For this review, take the finished solid that the model builds, in its own axes (mm). A direction names the side the tool comes from. Coordinates: 2 decimals unless noted, no trailing zeros. One line per item, written item: value. Start each with the question number.
1. Insertion check: pin 1 (1.7 mm diameter, centred on y = -1, z = 328.5, fed in from -X). The pin has a flat end and moves straight along its axis. Give the tip position at first contact, or say it passes through.
2. To check wall thickness, follow line 1 (Y direction, x = 0, z = 22.5); line 2 (Y direction, x = 0.25, z = 302.5); line 3 (Y direction, x = 4, z = 232). State the ranges of each line that lie inside material, in increasing order. Write a range as from..to.
3. For faces 5 (the face through (-3.9, 0, 28)), 6 (the face through (2, 2, 0)), 7 (the face through (3.9, 0, 28)), list the 3-axis set-ups (+Z, -Z, +X, -X, +Y, -Y) from which the entire face can be reached by the end or side of a thin tool; tool diameter is ignored.
4. The part is to be moulded in two halves that separate along Y. For faces 1 (the face through (0.057, -2.843, 56.541)), 2 (the face through (0, -3.9, 177)), 3 (the face through (0, 3.9, 177)), 4 (the face through (3.9, 0, 331)), say which applies: released by +Y, released by -Y, zero draft, split by the parting line, or undercut.
```python
from build123d import *

# Parameters (mm, degrees)
SKETCH_2_R          = 2.55
EXTRUDE_1_DEPTH     = 360
SKETCH_3_R          = 3
CUT_EXTRUDE_1_DEPTH = 361.693775937


with BuildPart() as part:
    # 草图2 → 凸台-拉伸1 (new body)
    with BuildSketch(Plane.XY):
        with BuildLine():
            Line((-3.9, 2.839339828), (-6.560660172, 5.5))
            Line((-6.560660172, 5.5), (-8.2, 5.5))
            Line((-8.2, 5.5), (-8.2, 3.1))
            Line((-8.2, 3.1), (-9.45, 3.1))
            Line((-9.45, 3.1), (-9.45, 3.65))
            Line((-9.45, 3.65), (-10, 3.65))
            Line((-10, 3.65), (-10, 8.5))
            ThreePointArc((-10, 8.5), (-9.560660172, 9.560660172), (-8.5, 10))
            Line((-8.5, 10), (-3.65, 10))
            Line((-3.65, 10), (-3.65, 9.45))
            Line((-3.65, 9.45), (-3.1, 9.45))
            Line((-3.1, 9.45), (-3.1, 8.2))
            Line((-3.1, 8.2), (-5.5, 8.2))
            Line((-5.5, 8.2), (-5.5, 6.560660172))
            Line((-5.5, 6.560660172), (-2.839339828, 3.9))
            Line((-2.839339828, 3.9), (2.839339828, 3.9))
            Line((2.839339828, 3.9), (5.5, 6.560660172))
            Line((5.5, 6.560660172), (5.5, 8.2))
            Line((5.5, 8.2), (3.1, 8.2))
            Line((3.1, 8.2), (3.1, 9.45))
            Line((3.1, 9.45), (3.65, 9.45))
            Line((3.65, 9.45), (3.65, 10))
            Line((3.65, 10), (8.5, 10))
            ThreePointArc((8.5, 10), (9.560660172, 9.560660172), (10, 8.5))
            Line((10, 8.5), (10, 3.65))
            Line((10, 3.65), (9.45, 3.65))
            Line((9.45, 3.65), (9.45, 3.1))
            Line((9.45, 3.1), (8.2, 3.1))
            Line((8.2, 3.1), (8.2, 5.5))
            Line((8.2, 5.5), (6.560660172, 5.5))
            Line((6.560660172, 5.5), (3.9, 2.839339828))
            Line((3.9, 2.839339828), (3.9, -2.839339828))
            Line((3.9, -2.839339828), (6.560660172, -5.5))
            Line((6.560660172, -5.5), (8.2, -5.5))
            Line((8.2, -5.5), (8.2, -3.1))
            Line((8.2, -3.1), (9.45, -3.1))
            Line((9.45, -3.1), (9.45, -3.65))
            Line((9.45, -3.65), (10, -3.65))
            Line((10, -3.65), (10, -8.5))
            ThreePointArc((10, -8.5), (9.560660172, -9.560660172), (8.5, -10))
            Line((8.5, -10), (3.65, -10))
            Line((3.65, -10), (3.65, -9.45))
            Line((3.65, -9.45), (3.1, -9.45))
            Line((3.1, -9.45), (3.1, -8.2))
            Line((3.1, -8.2), (5.5, -8.2))
            Line((5.5, -8.2), (5.5, -6.560660172))
            Line((5.5, -6.560660172), (2.839339828, -3.9))
            Line((2.839339828, -3.9), (-2.839339828, -3.9))
            Line((-2.839339828, -3.9), (-5.5, -6.560660172))
            Line((-5.5, -6.560660172), (-5.5, -8.2))
            Line((-5.5, -8.2), (-3.1, -8.2))
            Line((-3.1, -8.2), (-3.1, -9.45))
            Line((-3.1, -9.45), (-3.65, -9.45))
            Line((-3.65, -9.45), (-3.65, -10))
            Line((-3.65, -10), (-8.5, -10))
            ThreePointArc((-8.5, -10), (-9.560660172, -9.560660172), (-10, -8.5))
            Line((-10, -8.5), (-10, -3.65))
            Line((-10, -3.65), (-9.45, -3.65))
            Line((-9.45, -3.65), (-9.45, -3.1))
            Line((-9.45, -3.1), (-8.2, -3.1))
            Line((-8.2, -3.1), (-8.2, -5.5))
            Line((-8.2, -5.5), (-6.560660172, -5.5))
            Line((-6.560660172, -5.5), (-3.9, -2.839339828))
            Line((-3.9, -2.839339828), (-3.9, 2.839339828))
        make_face()
        with Locations(Location((0, 0, 0), (0, 0, 180))):
            Circle(SKETCH_2_R, mode=Mode.SUBTRACT)
    extrude(amount=EXTRUDE_1_DEPTH)

    # 草图3 → 切除-拉伸1 (cut, through all)
    with BuildSketch(Plane(origin=(10, 0, 0), x_dir=(0, 0, -1), z_dir=(1, 0, 0))):
        with Locations(Location((-57.5, 0, 0), (0, 0, 71.16400384))):
            Circle(SKETCH_3_R)
        with Locations(Location((-302.5, 0, 0), (0, 0, 108.835996159))):
            Circle(SKETCH_3_R)
    extrude(amount=-CUT_EXTRUDE_1_DEPTH, mode=Mode.SUBTRACT)


solid = part.part
```
Solutions:
1. pin 1: x = -3.9
2. line 1: -3.9..-2.55, 2.55..3.9
2. line 2: -3.9..-3, 3..3.9
2. line 3: -10..-8.2, -5.06..-2.94, 2.94..5.06, 8.2..10
3. face 5: +Z, -Z, -X
3. face 6: -Z, +X, -X, +Y, -Y
3. face 7: +Z, -Z, +X
4. face 1: undercut
4. face 2: released by -Y
4. face 3: released by +Y
4. face 4: undercut
